Design review of the part built by this model. Coordinates are the model's own, in mm. A direction names the side the tool comes from. Coordinates: 2 decimals unless noted, no trailing zeros. Write each loop counter-clockwise with the first axis right and the second up, starting at its lowest first coordinate (ties: lowest second). Pieces come first, ordered by that corner, then holes. Notation, with made-up numbers: (-5, 36.5) - (44, 36.5) arc R33 cw to (44, 65.5) - close; hole circle Ø5 at (19.5, -35.5). An arc over 180 degrees is marked (long way). Answer as CSV lines item,"result". Start each with the question number.
Q1. For line 1 along Y through (x, z) = (55, 6.25); line 2 along Y through (x, z) = (16.5, 5); line 3 along X through (y, z) = (-31, 4), list the stretches that pass through material, from the lowest coordinate up. Write a range as [from, to].
Q2. Machinability: for faces 1 (the face through (-28.5, -21.07, 5.07)), 2 (the face through (63, 37, 5)), which of the approach directions +Z, -Z, +X, -X, +Y, -Y give a long, thin tool a straight path to every point of the face, cutting with its end or side? Answer none if there is none.
Q3. Clearance check with a flat-ended pin moving along its axis: pin 1 (6 mm diameter, centred on x = 55, y = 30, fed in from +Z). State where the tip first meets the part, or that it passes through.
Q4. Mouldability with a two-part tool opening along X and no side actions: class faces 3 (the face through (-1, 27, 0)), 4 (the face through (-62, 38, 5)), 5 (the face through (-51.7, 30.1, 4.9)) as pulls with the +X half, pulls with the -X half, needs draft (parallel to the pull), parting line crosses it, or undercut.
Q5. We need section C-C (z = 3). Write out the cut boundary in (x, y).
Q6. We need section A-A (y = -14). Write out the cut boundary in (x, z), plus the area to 3 significant figures.
Q7. We need section B-B (x = -1). Write out the cut boundary in (y, z), plus the area to 3 significant figures.
Q8. We need section D-D (y = -30). Write out the cut boundary in (x, z).
from build123d import *

# Parameters (mm, degrees)
F0_W     = 130
F0_H     = 80
F0_W_2   = 60
F0_H_2   = 45
F1_DEPTH = 10
F3_R     = 5
F4_SIZE  = 5
F5_D     = 6.6
F5_DEPTH = 20
F5_TIP   = 1.9828400428


with BuildPart() as f1:
    # F0 (on Top) → F1 (new body)
    with BuildSketch(Plane.XY):
        Rectangle(F0_W, F0_H)
        Rectangle(F0_W_2, F0_H_2, mode=Mode.SUBTRACT)
    extrude(amount=F1_DEPTH)

    # F3
    f3_edges = [f1.edges().sort_by_distance(p)[0] for p in [
        (-30, 22.5, 5),
        (-30, -22.5, 5),
        (30, -22.5, 5),
        (30, 22.5, 5),
    ]]
    fillet(f3_edges, radius=F3_R)

    # F4
    f4_edges = [f1.edges().sort_by_distance(p)[0] for p in [
        (-65, -40, 5),
        (-65, 40, 5),
        (65, -40, 5),
        (65, 40, 5),
    ]]
    chamfer(f4_edges, length=F4_SIZE)

    # F5
    with Locations(Plane.XY.offset(10)):
        with Locations((-55, 30), (-55, -30), (55, -30), (55, 30)):
            Hole(F5_D / 2, depth=F5_DEPTH)
            with Locations((0, 0, -(F5_DEPTH + F5_TIP / 2))):  # 118° drill point
                Cone(0, F5_D / 2, F5_TIP, mode=Mode.SUBTRACT)


solid = f1.part
Results list:
1,line 1,"y = [-40, -33.3], [-26.7, 26.7], [33.3, 40]"
1,line 2,"y = [-40, -22.5], [22.5, 40]"
1,line 3,"x = [-65, -58.14], [-51.86, 51.86], [58.14, 65]"
2,face 1,"+Z, -Z"
2,face 2,"+Z, -Z, +X, +Y"
3,pin 1,"passes through"
4,face 3,"needs draft"
4,face 4,"pulls with the -X half"
4,face 5,"undercut"
5,outline,"(-65, -35) - (-60, -40) - (60, -40) - (65, -35) - (65, 35) - (60, 40) - (-60, 40) - (-65, 35) - close; hole circle Ø6.6 at (-55, -30); hole circle Ø6.6 at (-55, 30); hole (-30, -17.5) arc R5 ccw to (-25, -22.5) - (25, -22.5) arc R5 ccw to (30, -17.5) - (30, 17.5) arc R5 ccw to (25, 22.5) - (-25, 22.5) arc R5 ccw to (-30, 17.5) - close; hole circle Ø6.6 at (55, -30); hole circle Ø6.6 at (55, 30)"
6,outline,"(-65, 0) - (-30, 0) - (-30, 10) - (-65, 10) - close; (30, 0) - (65, 0) - (65, 10) - (30, 10) - close"
6,area,"700 mm2"
7,outline,"(-40, 0) - (-22.5, 0) - (-22.5, 10) - (-40, 10) - close; (22.5, 0) - (40, 0) - (40, 10) - (22.5, 10) - close"
7,area,"350 mm2"
8,outline,"(-65, 0) - (-58.3, 0) - (-58.3, 10) - (-65, 10) - close; (-51.7, 0) - (51.7, 0) - (51.7, 10) - (-51.7, 10) - close; (58.3, 0) - (65, 0) - (65, 10) - (58.3, 10) - close"
